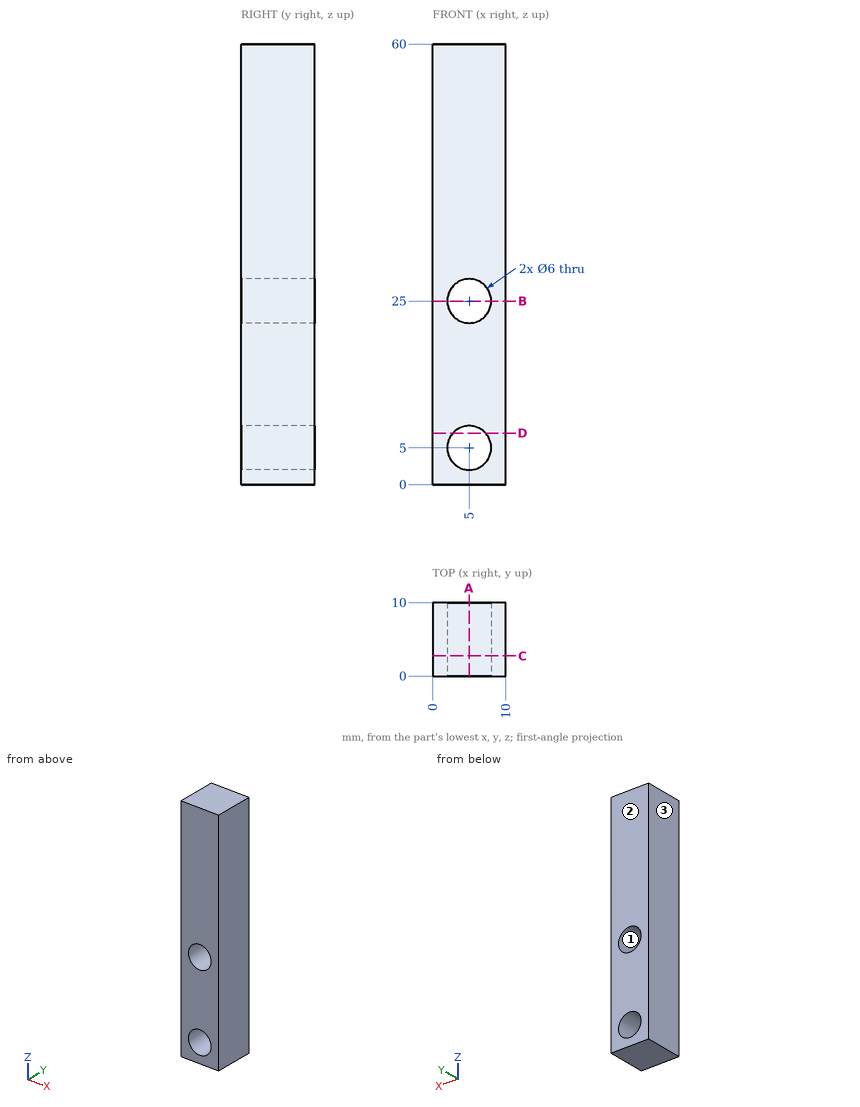
Print and shaded views of the part. All mm, measured from the part's lowest x, y and z. Round coordinates to 2 decimals unless told otherwise and drop trailing zeros. Loops run counter-clockwise (first coordinate to the right, second up) from the corner with the lowest first, then second, coordinate; pieces in that order, holes last. Notation, with made-up numbers: (-8.75, -31) -> (5.25, -31) arc R29 ccw to (5.25, -10) -> close; hole circle Ø8 at (-4.5, 19). An arc over 180 degrees is marked (long way). Use CSV: the item, a comma, the result in double quotes. Start each with the question number.
1) Cut at C-C, the plane y = 2.75. Write the cut outline in (x, z), plus the area to 3 significant figures.
2) Cut at D-D, the plane z = 7. Write the cut outline in (x, y), plus the area to 3 significant figures.
3) Pull direction X, two halves, no side cores. Call the marked faces 1, 2 and 3: +X half, -X half, draft (parallel to the pull), parting line (faces both ways), or undercut.
4) Wall check: L1, parallel to Z at x = 5, y = 6; L2, parallel to X at y = 2.25, z = 5; L3, parallel to Z at x = 2.5, y = 3.25. Give the ranges that are in metal, low to high. Write a range as [from, to].
5) Cut at B-B, the plane z = 25. Write the cut outline in (x, y), plus the area to 3 significant figures.
6) Cut at A-A, the plane x = 5. Write the cut outline in (y, z).
7) Drop a flat-ended pin along its axis: P1, Ø5.5, axis at x = 5, z = 5, coming from the +Y side. Give the stop position or say it passes through.
Determined:
1,outline,"(0, 0) -> (10, 0) -> (10, 60) -> (0, 60) -> close; hole circle Ø6 at (5, 5); hole circle Ø6 at (5, 25)"
1,area,"543 mm2"
2,outline,"(0, 0) -> (2.76, 0) -> (2.76, 10) -> (0, 10) -> close; (7.24, 0) -> (10, 0) -> (10, 10) -> (7.24, 10) -> close"
2,area,"55.3 mm2"
3,face 1,"undercut"
3,face 2,"draft"
3,face 3,"-X half"
4,L1,"z = [0, 2], [8, 22], [28, 60]"
4,L2,"x = [0, 2], [8, 10]"
4,L3,"z = [0, 3.34], [6.66, 23.34], [26.66, 60]"
5,outline,"(0, 0) -> (2, 0) -> (2, 10) -> (0, 10) -> close; (8, 0) -> (10, 0) -> (10, 10) -> (8, 10) -> close"
5,area,"40.0 mm2"
6,outline,"(0, 0) -> (10, 0) -> (10, 2) -> (0, 2) -> close; (0, 8) -> (10, 8) -> (10, 22) -> (0, 22) -> close; (0, 28) -> (10, 28) -> (10, 60) -> (0, 60) -> close"
7,P1,"passes through"
